For this review, take the finished solid that the model builds, in its own axes (mm). Round coordinates to 2 decimals unless told otherwise and drop trailing zeros. Write each loop counter-clockwise with the first axis right and the second up, starting at its lowest first coordinate (ties: lowest second). Pieces come first, ordered by that corner, then holes. Notation, with made-up numbers: (0.5, -30.75) -> (30.5, -30.75) arc R25 ccw to (30.5, 0.25) -> close; hole circle Ø2 at (46, -15). An arc over 180 degrees is marked (long way). Answer as CSV lines item,"result". Start each with the question number.
Item 1: Wall thickness on probe 1 along Z at (x, y) = (-17.5, 59.85); probe 2 along X at (y, z) = (59.8, -17.5); probe 3 along Z at (x, y) = (16, 59.8): over which ranges is each line inside the solid? List them lowest first. Write a range as from..to.
Item 2: Take a section at A-A on y = 59.85. Give the boundary of the cut face in (x, z).
Item 3: Mouldability with a two-part tool opening along Z and no side actions: class faces 1 (the flat face through (0, 59.5, 0)), 2 (the cylindrical face through (-21.009, 59.754, 21.074)), 3 (the cylindrical face through (-21.009, 59.754, -21.074)), 4 (the cylindrical face through (19.123, 59.754, 17.858)) as +Z half, -Z half, draft (parallel to the pull), parting line (faces both ways), or undercut.
```python
from build123d import *

# Parameters (mm, degrees)
SKETCH1_W                                  = 45.025374044
SKETCH1_H                                  = 45
BOSS_EXTRUDE1_DEPTH                        = 60
FILLET3_R                                  = 5
FILLET4_R                                  = 5
FILLET7_R                                  = 5
FILLET8_R                                  = 5
SKETCH9_R                                  = 1.65
CUT_EXTRUDE6_DEPTH                         = 5
MIRROR2_AT_THE_SECOND_PLANE_COPY_1_SKETC_R = 1.65
MIRROR2_AT_THE_SECOND_PLANE_COPY_1_DEPTH   = 5
SKETCH10_W                                 = 54.362738508
SKETCH10_H                                 = 47.512908914
CUT_EXTRUDE7_DEPTH                         = 59.5


with BuildPart() as part:
    # Sketch1 → Boss-Extrude1 (new body)
    with BuildSketch(Plane(origin=(0, 0, 0), x_dir=(1, 0, 0), z_dir=(0, 1, 0))):
        Rectangle(SKETCH1_W, SKETCH1_H)
    extrude(amount=BOSS_EXTRUDE1_DEPTH)

    # Fillet3
    fillet3_edges = [part.edges().sort_by_distance(p)[0] for p in [
        (22.512687022, 30, -22.5),
    ]]
    fillet(fillet3_edges, radius=FILLET3_R)

    # Fillet4
    fillet4_edges = [part.edges().sort_by_distance(p)[0] for p in [
        (-22.512687022, 30, -22.5),
    ]]
    fillet(fillet4_edges, radius=FILLET4_R)

    # Fillet7
    fillet7_edges = [part.edges().sort_by_distance(p)[0] for p in [
        (22.512687022, 30, 22.5),
    ]]
    fillet(fillet7_edges, radius=FILLET7_R)

    # Fillet8
    fillet8_edges = [part.edges().sort_by_distance(p)[0] for p in [
        (-22.512687022, 30, 22.5),
    ]]
    fillet(fillet8_edges, radius=FILLET8_R)

    # Sketch9 → Cut-Extrude6 (cut)
    with BuildSketch(Plane(origin=(0, 60, 0), x_dir=(1, 0, 0), z_dir=(0, 1, 0))):
        with Locations(Location((-17.512687022, 17.5, 0), (0, 0, 270))):
            Circle(SKETCH9_R)
    cut_extrude6 = extrude(amount=-CUT_EXTRUDE6_DEPTH, mode=Mode.SUBTRACT)

    # Mirror2: Cut-Extrude6 across plane
    add(cut_extrude6.mirror(Plane(origin=(0, 0, 0), x_dir=(0, 0, 1), z_dir=(1, 0, 0))), mode=Mode.SUBTRACT)

    # Mirror2 at the second plane: Cut-Extrude6 across plane
    add(cut_extrude6.mirror(Plane.XY), mode=Mode.SUBTRACT)

    # Mirror2 at the second plane copy 1 sketc → Mirror2 at the second plane copy 1 (cut)
    with BuildSketch(Plane(origin=(0, 60, 0), x_dir=(-1, 0, 0), z_dir=(0, 1, 0))):
        with Locations(Location((-17.512687022, 17.5, 0), (0, 0, 270))):
            Circle(MIRROR2_AT_THE_SECOND_PLANE_COPY_1_SKETC_R)
    extrude(amount=-MIRROR2_AT_THE_SECOND_PLANE_COPY_1_DEPTH, mode=Mode.SUBTRACT)

    # Sketch10 → Cut-Extrude7 (cut)
    with BuildSketch(Plane.XZ):
        Rectangle(SKETCH10_W, SKETCH10_H)
    extrude(amount=-CUT_EXTRUDE7_DEPTH, mode=Mode.SUBTRACT)


solid = part.part
```
Output values:
1,probe 1,"z = -22.5..-19.15, -15.85..15.85, 19.15..22.5"
1,probe 2,"x = -22.51..-19.16, -15.86..15.86, 19.16..22.51"
1,probe 3,"z = -22.5..-18.16, -16.84..16.84, 18.16..22.5"
2,outline,"(-22.51, -17.5) arc R5 ccw to (-17.51, -22.5) -> (17.51, -22.5) arc R5 ccw to (22.51, -17.5) -> (22.51, 17.5) arc R5 ccw to (17.51, 22.5) -> (-17.51, 22.5) arc R5 ccw to (-22.51, 17.5) -> close; hole circle Ø3.3 at (-17.51, -17.5); hole circle Ø3.3 at (-17.51, 17.5); hole circle Ø3.3 at (17.51, -17.5); hole circle Ø3.3 at (17.51, 17.5)"
3,face 1,"draft"
3,face 2,"+Z half"
3,face 3,"-Z half"
3,face 4,"undercut"
